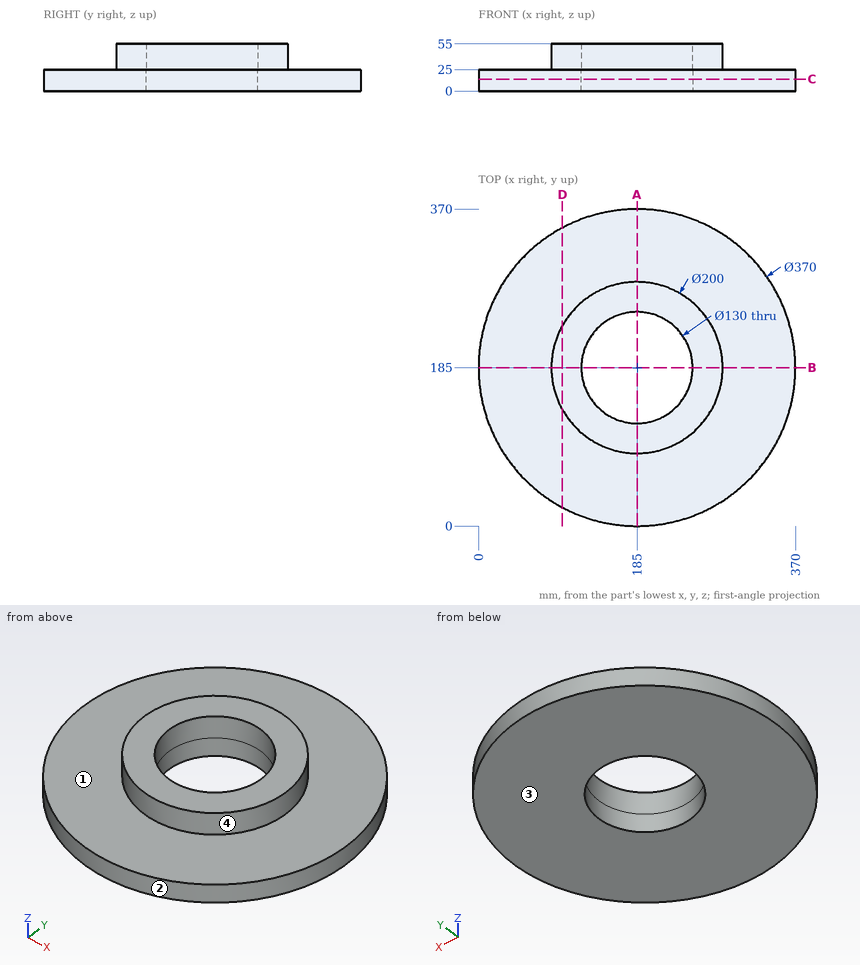
Design review of the part shown in the three views and the two pictorial views. Dimensions are in mm from the part's minimum x, y and z. A direction names the side the tool comes from. Give positions to 0.01 mm unless a question says otherwise; leave off trailing zeros. Loops run counter-clockwise (first coordinate to the right, second up) from the corner with the lowest first, then second, coordinate; pieces in that order, holes last. Notation, with made-up numbers: M -19,50.5 L 15,50.5 A32 ccw 15,88.5 Z; hole C 55.5,72 d4. An arc over 180 degrees is marked long. Answer as a JSON object with one key per item and string values. Group by question number.
Q1. For probe 1 along Y at (x, z) = (185, 34.25); probe 2 along Z at (x, y) = (128, 79); probe 3 along Y at (x, z) = (185, 13.25), list the stretches that pass through material, from the lowest coordinate up. Write a range as [from, to].
Q2. Mouldability with a two-part tool opening along Y and no side actions: class the marked faces 3 and 4 as +Y half, -Y half, draft (parallel to the pull), parting line (faces both ways), or undercut.
Q3. Add section C-C on z = 14. Give the boundary of the cut face in (x, y).
Q4. Add section D-D on x = 98. Give the boundary of the cut face in (y, z), and give its area (3 significant figures).
Q5. Insertion check: P1, Ø2, axis at y = 215.5, z = 13.5, coming from the -X side; P2, Ø8, axis at x = 213.5, y = 302.5, coming from the +Z side; P3, Ø4, axis at x = 199, z = 6.5, coming from the +Y side. Each pin has a flat end and moves straight along its axis. Give the tip position at first contact, or say it passes through.
Q6. Tool access review of the marked faces 1 and 2: name each direction out of +Z, -Z, +X, -X, +Y, -Y from which nothing blocks a thin tool from reaching the whole face with its end or side.
Q7. Add section A-A on x = 185. Give the boundary of the cut face in (y, z).
Checked values:
{
 "1": {"probe 1": "[85, 120], [250, 285]", "probe 2": "[0, 25]", "probe 3": "[0, 120], [250, 370]"},
 "2": {"face 3": "draft", "face 4": "parting line"},
 "3": {"outline": "C 185,185 d370; hole C 185,185 d130"},
 "4": {"outline": "M 21.73,0 L 348.27,0 L 348.27,25 L 234.31,25 L 234.31,55 L 135.69,55 L 135.69,25 L 21.73,25 Z", "area": "11,100 mm²"},
 "5": {"P1": "x = 2.37", "P2": "z = 25", "P3": "y = 369.61"},
 "6": {"face 1": "+Z", "face 2": "+Z, -Z"},
 "7": {"outline": "M 0,0 L 120,0 L 120,55 L 85,55 L 85,25 L 0,25 Z; M 250,0 L 370,0 L 370,25 L 285,25 L 285,55 L 250,55 Z"}
}
